Build history of the part. All positions in model axes, mm. Round coordinates to 2 decimals unless told otherwise and drop trailing zeros. Write each loop counter-clockwise with the first axis right and the second up, starting at its lowest first coordinate (ties: lowest second). Pieces come first, ordered by that corner, then holes. Notation, with made-up numbers: (84, 20.5) - (137, 20.5) arc R19 ccw to (137, 42.5) - close; hole circle Ø2 at (-14, -7.75). An arc over 180 degrees is marked (long way). One line per question, with ' | ' between items.
from build123d import *

# Parameters (mm, degrees)
SKETCH_1_R          = 20
EXTRUDE_1_DEPTH     = 4
SKETCH_2_R          = 9.5
CUT_EXTRUDE_1_DEPTH = 41.509258201
SKETCH_4_R          = 1.5
CUT_EXTRUDE_2_DEPTH = 41.509258201


with BuildPart() as part:
    # 草图1 → 凸台-拉伸1 (new body)
    with BuildSketch(Plane.XY):
        Circle(SKETCH_1_R)
        with BuildLine():
            ThreePointArc((20, 0), (0, -20), (-20, 0))
            Line((-20, 0), (-20, -35))
            Line((-20, -35), (20, -35))
            Line((20, -35), (20, 0))
        make_face()
    extrude(amount=EXTRUDE_1_DEPTH)

    # 草图2 → 切除-拉伸1 (cut, through all)
    with BuildSketch(Plane.XY.offset(4)):
        Circle(SKETCH_2_R)
    extrude(amount=-CUT_EXTRUDE_1_DEPTH, mode=Mode.SUBTRACT)

    # 草图4 → 切除-拉伸2 (cut, through all)
    with BuildSketch(Plane.XY.offset(4)):
        with Locations((-15, -26)):
            Circle(SKETCH_4_R)
        with Locations(Location((15, -26, 0), (0, 0, 180))):
            Circle(SKETCH_4_R)
    extrude(amount=-CUT_EXTRUDE_2_DEPTH, mode=Mode.SUBTRACT)


solid = part.part
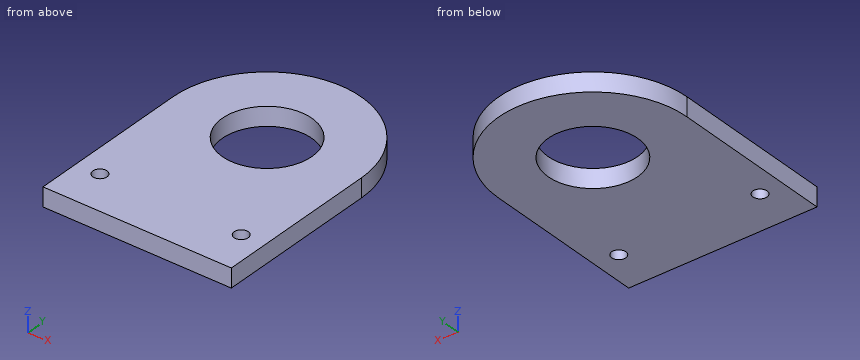
Q1. Saw through at D-D, the plane y = 1.5. List the corners of the cut face in (x, z), then the cut area to 3 significant figures.
Found:
outline: (-19.94, 0) - (-9.38, 0) - (-9.38, 4) - (-19.94, 4) - close; (9.38, 0) - (19.94, 0) - (19.94, 4) - (9.38, 4) - close | area: 84.5 mm^2
Q2. Saw through at A-A, the plane y = -26. List the corners of the cut face in (x, z), then the cut area to 3 significant figures.
Found:
outline: (-20, 0) - (-16.5, 0) - (-16.5, 4) - (-20, 4) - close; (-13.5, 0) - (13.5, 0) - (13.5, 4) - (-13.5, 4) - close; (16.5, 0) - (20, 0) - (20, 4) - (16.5, 4) - close | area: 136 mm^2
Q3. Drill centre lines: L1, parallel to Y at x = 0, z = 0.8; L2, parallel to Y at x = 15, z = 1; L3, parallel to Y at x = 17, z = 1. Where is each one in solid material? Low to high. Write a range as from..to.
Found:
L1: -35..-9.5, 9.5..20 | L2: -35..-27.5, -24.5..13.23 | L3: -35..10.54
Q4. Drop flat-ended pins along their axis: pin 1 (1 mm diameter, centred on y = 14, z = 3, fed in from +X); pin 2 (1 mm diameter, centred on y = 1.5, z = 2, fed in from -X) (3 decimals). Give the stop position or say it passes through.
Found:
pin 1: x = 14.76 | pin 2: x = -19.975
Q5. Saw through at B-B, the plane z = 2.1. List the corners of the cut face in (x, y), then the cut area to 3 significant figures.
Found:
outline: (-20, -35) - (20, -35) - (20, 0) arc R20 ccw to (-20, 0) - close; hole circle Ø3 at (-15, -26); hole circle Ø19 at (0, 0); hole circle Ø3 at (15, -26) | area: 1,730 mm^2
Q6. Saw through at C-C, the plane x = 0. List the corners of the cut face in (y, z), then the cut area to 3 significant figures.
Found:
outline: (-35, 0) - (-9.5, 0) - (-9.5, 4) - (-35, 4) - close; (9.5, 0) - (20, 0) - (20, 4) - (9.5, 4) - close | area: 144 mm^2
